Geometry check sheet. Reference: the model listing, model coordinates, mm. A direction names the side the tool comes from. Coordinates: 2 decimals unless noted, no trailing zeros. Write each loop counter-clockwise with the first axis right and the second up, starting at its lowest first coordinate (ties: lowest second). Pieces come first, ordered by that corner, then holes. Notation, with made-up numbers: M 0,-12 L 7,-12 A10 ccw 7,7 Z; hole C -25.75,-20 d5. An arc over 180 degrees is marked long. Write each question's results on one line, items separated by ' | '.
```python
from build123d import *

# Parameters (mm, degrees)
SKETCH_1_W             = 100
SKETCH_1_H             = 2
REVOLVE_1_ANGLE        = 180
SKETCH_3_W             = 3
SKETCH_3_H             = 10
REVOLVE_2_ANGLE        = 180
FILLET_1_R             = 5
FILLET_1_OF_MIRROR_1_R = 5


with BuildPart() as part:
    # ｽｹｯﾁ1 → 回転1 (revolve)
    with BuildSketch(Plane.XY):
        with Locations((0, 99)):
            Rectangle(SKETCH_1_W, SKETCH_1_H)
    revolve(axis=Axis((-50, 0, 0), (-1, 0, 0)), revolution_arc=REVOLVE_1_ANGLE)

    # ｽｹｯﾁ3 → 回転2 (revolve)
    with BuildSketch(Plane.XY):
        with Locations((51.5, 95)):
            Rectangle(SKETCH_3_W, SKETCH_3_H)
    revolve_2 = revolve(axis=Axis((-50, 0, 0), (-1, 0, 0)), revolution_arc=REVOLVE_2_ANGLE)

    # ﾌｨﾚｯﾄ1
    fillet_1_edges = [part.edges().sort_by_distance(p)[0] for p in [
        (50, 0, -98),
    ]]
    fillet(fillet_1_edges, radius=FILLET_1_R)

    # ﾐﾗｰ1: 回転2 across plane
    add(revolve_2.mirror(Plane(origin=(0, 0, 0), x_dir=(0, 0, 1), z_dir=(1, 0, 0))))

    # ﾌｨﾚｯﾄ1 of ﾐﾗｰ1
    fillet_1_of_mirror_1_edges = [part.edges().sort_by_distance(p)[0] for p in [
        (-50, 0, -98),
    ]]
    fillet(fillet_1_of_mirror_1_edges, radius=FILLET_1_OF_MIRROR_1_R)


solid = part.part
```
Q1. Scan lines: probe 1 along X at (y, z) = (80, -43); probe 2 along Y at (x, z) = (-37, -22.5); probe 3 along Y at (x, z) = (22, -72). Record each from-to range of solid material in increasing order.
Geometry check:
probe 1: x = -53 to -50, 50 to 53 | probe 2: y = -97.44 to -95.38, 95.38 to 97.44 | probe 3: y = -69.4 to -66.48, 66.48 to 69.4
Q2. Depth check by flat-ended pin: P1, Ø1, axis at x = -10.5, y = -74, coming from the +Z side; P2, Ø5, axis at x = -19.5, y = -73.5, coming from the +Z side; P3, Ø6, axis at x = -32.5, z = -72.5, coming from the -Y side. Enter the tip coordinate at first touch or a pass-through.
Geometry check:
P1: stops at z = -63.67 | P2: stops at z = -61.87 | P3: stops at y = -71.9
Q3. Access from +Z, -Z, +X, -X, +Y, -Y to the whole of each face (thin tool, end or side, straight path). Record for faces 5 (the cylindrical face through (51.52, 1.98, -89.98)), 6 (the flat face through (50, 21, -88)).
Geometry check:
face 5: +Z, +X, -X | face 6: +Z
Q4. Sectioned sample at B-B on x = -23. Record the cut outline in (y, z).
Geometry check:
outline: M -100,0 A100 ccw 100,0 L 98,0 A98 cw -98,0 Z
Q5. Mould release check, pull along X, two halves, no side actions. Record for faces 1 (the cylindrical face through (-0.742, 2.199, -99.976)), 2 (the flat face through (-50, 21, -88)), 3 (the flat face through (53, 0, -91)), 4 (the cylindrical face through (0.63, 2.155, -97.976)): pulls with the +X half, pulls with the -X half, needs draft (parallel to the pull), parting line crosses it, or undercut.
Geometry check:
face 1: needs draft | face 2: undercut | face 3: pulls with the +X half | face 4: undercut
Q6. Sectioned sample at A-A on y = 0. Record the cut outline in (x, z), and give its area (3 significant figures).
Geometry check:
outline: M -53,-100 L 53,-100 L 53,-90 L 50,-90 L 50,-93 A5 cw 45,-98 L -45,-98 A5 cw -50,-93 L -50,-90 L -53,-90 Z | area: 271 mm2
